from build123d import *

# Parameters (mm, degrees)
BOSS_EXTRUDE1_DEPTH = 95.25
CUT_EXTRUDE1_DEPTH  = 9
SKETCH5_R           = 1.25
CUT_EXTRUDE2_DEPTH  = 3


with BuildPart() as part:
    # Sketch1 → Boss-Extrude1 (new body)
    with BuildSketch(Plane.XY):
        Polygon((0, 0), (-111.31, 0), (-111.31, -73.29), (-115.41, -73.29), (-115.41, -114.29), (-111.31, -114.29), (-111.31, -137.31), (-118.84, -137.31), (-118.84, -140.99), (-109.31, -140.99), (-109.31, -150.62), (-127.92, -150.62), (-127.92, 15.09), (0, 15.09), (0, 10.99), (-17.1, 10.99), (-17.1, 4.1), (0, 4.1), align=None)
    extrude(amount=BOSS_EXTRUDE1_DEPTH)

    # Sketch4 → Cut-Extrude1 (cut)
    with BuildSketch(Plane(origin=(0, 0, 0), x_dir=(-1, 0, 0), z_dir=(0, 0, -1))):
        Polygon((111.31, 0), (0, 0), (0, 10.99), (44.73, 10.99), (44.73, 15.09), (111.31, 15.09), align=None)
    extrude(amount=-CUT_EXTRUDE1_DEPTH, mode=Mode.SUBTRACT)

    # Sketch5 → Cut-Extrude2 (cut)
    with BuildSketch(Plane(origin=(-115.41, 0, 0), x_dir=(0, 0, -1), z_dir=(1, 0, 0))):
        with Locations((-43.46, -105.21)):
            Circle(SKETCH5_R)
        with Locations((-61.46, -85.71)):
            Circle(SKETCH5_R)
    extrude(amount=-CUT_EXTRUDE2_DEPTH, mode=Mode.SUBTRACT)


solid = part.part
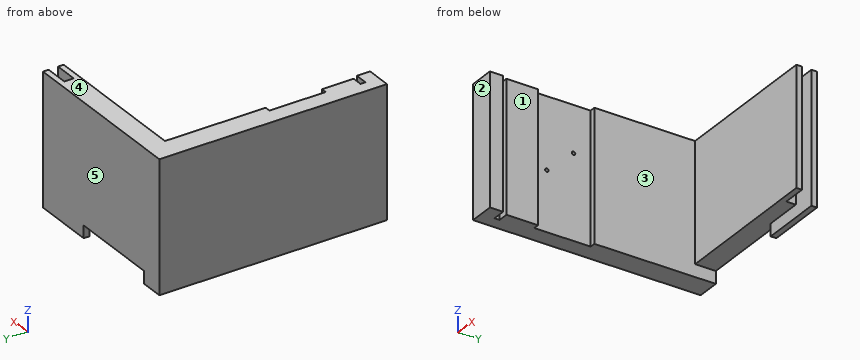
Read the model definition and answer for the solid it produces. Units are mm, in the model's axes. Face numbers are marked on the shaded views. A direction names the side the tool comes from. Round coordinates to 2 decimals unless told otherwise and drop trailing zeros. Loops run counter-clockwise (first coordinate to the right, second up) from the corner with the lowest first, then second, coordinate; pieces in that order, holes last.
Q1. Consider probe 1 along Y at (x, z) = (-116.85, 61.46); probe 2 along Y at (x, z) = (-117.3, 43.46); probe 3 along Z at (x, y) = (-117.5, -85.71). Determine where each line is inside the solid, lowest interval first.
Q2. Determine the mould class of the marked faces 3, 4 and 5 for opening direction Y: released by +Y, released by -Y, zero draft, split by the parting line, or undercut.
Q3. Each of these flat-tipped pins is pushed along its axis until it touches: pin 1 (4.5 mm diameter, centred on x = -71, y = 5, fed in from -Z); pin 2 (3 mm diameter, centred on y = -85.71, z = 61.46, fed in from +X); pin 3 (1.2 mm diameter, centred on y = -85.5, z = 61.5, fed in from +X). Where does it stop, or does it pass through?
Q4. Which of the six approach directions +Z, -Z, +X, -X, +Y, -Y give full straight-line access (tool end or side, diameter ignored) to the marked faces 1 and 2?
Q5. Section C-C on x = -75 is taken. Write down the section's boundary in (y, z), and give its area (3 significant figures).
Q6. Section A-A on z = 33 is taken. Write down the section's boundary in (x, y).
Q7. Section B-B on y = -126 is taken. Write down the section's boundary in (x, z), and give its area (3 significant figures).
Output:
1. probe 1: y = -150.62 to -140.99, -137.31 to -86.96, -84.46 to 15.09
1. probe 2: y = -150.62 to -140.99, -137.31 to -106.46, -103.96 to 15.09
1. probe 3: z = 0 to 60.21, 62.71 to 95.25
2. face 3: undercut
2. face 4: zero draft
2. face 5: released by +Y
3. pin 1: stops at z = 9
3. pin 2: stops at x = -115.41
3. pin 3: stops at x = -118.41
4. face 1: +Z, -Z, +X
4. face 2: +Z, -Z, +X, -X, -Y
5. outline: (0, 9) - (15.09, 9) - (15.09, 95.25) - (0, 95.25) - close
5. area: 1,300 mm2
6. outline: (-127.92, -150.62) - (-109.31, -150.62) - (-109.31, -140.99) - (-118.84, -140.99) - (-118.84, -137.31) - (-111.31, -137.31) - (-111.31, -114.29) - (-115.41, -114.29) - (-115.41, -73.29) - (-111.31, -73.29) - (-111.31, 0) - (0, 0) - (0, 4.1) - (-17.1, 4.1) - (-17.1, 10.99) - (0, 10.99) - (0, 15.09) - (-127.92, 15.09) - close
7. outline: (-127.92, 0) - (-111.31, 0) - (-111.31, 95.25) - (-127.92, 95.25) - close
7. area: 1,580 mm2
